Autodesk Inventor part; units mm, degrees
ref_plane "YZ Plane" through (0, 0, 0) normal (1, 0, 0) x (0, 1, 0)
ref_plane "XZ Plane" through (0, 0, 0) normal (0, 1, 0) x (-1, 0, 0)
ref_plane "XY Plane" through (0, 0, 0) normal (0, 0, 1) x (1, 0, 0)
sketch "Sketch1" plane through (0, 0, 0) normal (0, 0, 1) x (1, 0, 0)
  line L0 (0, 0) -> (0, 81.958)
  line L1 (0, 0) -> (0, -81.958)
  line L2 (0, -81.958) -> (-10, -81.958)
  line L3 (-5, -81.958) -> (-5, -67.708) construction
  line L4 (-5, -67.708) -> (-5, -58.708) construction
  line L5 (-10, -81.958) -> (-10, -58.708)
  line L6 (-10, -58.708) -> (0, -58.708)
  line L7 (0, 81.958) -> (-10, 81.958)
  line L8 (-5, 81.958) -> (-5, 66.21) construction
  line L9 (-5, 66.21) -> (-5, 20.031) construction
  line L10 (-5, 20.031) -> (-5, 11.031) construction
  line L11 (-10, 81.958) -> (-10, 11.031)
  line L12 (-10, 11.031) -> (0, 11.031)
  line L13 (0, -58.708) -> (-2, -58.708)
  line L14 (-2, -58.708) -> (-2, 11.031)
  line L15 (0, -81.958) -> (8, -81.958)
  line L16 (8, -81.958) -> (8, 81.958)
  line L17 (8, 81.958) -> (0, 81.958)
  line L18 (0, 81.958) -> (0, -81.958)
  dimension "d0" = 81.958
  dimension "d2" = 163.916
  dimension "d3" = 10
  dimension "d4" = 14.25
  dimension "d5" = 9
  dimension "d6" = 15.748
  dimension "d7" = 46.179
  dimension "d8" = 9
  dimension "d9" = 2
  dimension "d10" = 8
extrude "Extrusion1" add sketch "Sketch1" along normal blind 7
sketch "Sketch2" plane through (0, 0, 0) normal (0, 0, -1) x (-1, 0, 0)
  line L0 (10, 81.958) -> (10, 11.031) construction
  line L1 (10, 46.4945) -> (0, 46.4945) construction
  line L2 (-8, 81.958) -> (10, 81.958)
  line L3 (0, 81.958) -> (-50, 81.958)
  line L4 (-50, 81.958) -> (-50, -81.958)
  line L5 (-50, -81.958) -> (0, -81.958)
  line L6 (0, -81.958) -> (0, 81.958)
  line L7 (-35.1508, -57.5) -> (-20.1508, -57.5)
  line L8 (-20.1508, -57.5) -> (-20.1508, 57.5)
  line L9 (-20.1508, 57.5) -> (-35.1508, 57.5)
  line L10 (-35.1508, 57.5) -> (-35.1508, -57.5)
  line L11 (-35.1508, -57.5) -> (-20.1508, 57.5) construction
  line L12 (-20.1508, -57.5) -> (-35.1508, 57.5) construction
  point P0 (0, 0)
  point P1 (-27.6508, 0)
  dimension "d13" = 10
  dimension "d14" = 50
  dimension "d15" = 15
  dimension "d16" = 115
extrude "Extrusion2" add sketch "Sketch2" along normal blind 9
sketch "Sketch3" plane through (-10, -81.958, 7) normal (0, -1, 0) x (1, 0, 0)
  line L0 (60, -7) -> (18, -7)
  line L1 (60, -7) -> (60, 5)
  line L2 (0, 0) -> (18, 0)
  line L3 (18, 5) -> (18, 0)
  line L4 (60, 5) -> (39, -7)
  line L5 (18, 5) -> (39, -7)
  line L6 (18, -7) -> (18, 0)
  line L7 (18, 0) -> (18, -7)
  point P0 (10, -7)
  dimension "d19" = 12
extrude "Extrusion3" add sketch "Sketch3" against normal up to surface (24.458 mm away)
mirror "Mirror1" about plane through (0, 0, 0) normal (0, 1, 0) of "Extrusion3"
sketch "Sketch4" plane through (0, 0, 7) normal (0, 0, 1) x (1, 0, 0)
  line L0 (-5, -81.958) -> (-5, -67.708) construction
  line L1 (-5, 81.958) -> (-5, 66.21) construction
  line L2 (-5, 66.21) -> (-5, 20.031) construction
  circle A0 centre (-5, -67.708) radius 1.65
  circle A1 centre (-5, 20.031) radius 1.65
  circle A2 centre (-5, 66.21) radius 1.65
  point P0 (0, 0)
  dimension "d22" = 14.25
  dimension "d23" = 46.179
  dimension "d24" = 15.748
  dimension "d25" = 3.3
extrude "Extrusion4" cut sketch "Sketch4" against normal up to surface (7 mm away)
sketch "Sketch5" plane through (0, 0, 7) normal (0, 0, 1) x (1, 0, 0)
  circle A0 centre (-5, -67.708) radius 1.65
  circle A1 centre (-5, -67.708) radius 2.65
  circle A2 centre (-5, 20.031) radius 1.65
  circle A3 centre (-5, 20.031) radius 2.65
  circle A4 centre (-5, 66.21) radius 1.65
  circle A5 centre (-5, 66.21) radius 2.65
  point P0 (0, 0)
  dimension "d28" = 5.3
extrude "Extrusion5" cut sketch "Sketch5" against normal blind 6 contours A0 | A1 | A2 | A3 | A4 | A5
properties part number "Base Extension 2"
Read the model definition and answer for the solid it produces. Units are mm, in the model's axes. A direction names the side the tool comes from. Round coordinates to 2 decimals unless told otherwise and drop trailing zeros. Write each loop counter-clockwise with the first axis right and the second up, starting at its lowest first coordinate (ties: lowest second). Pieces come first, ordered by that corner, then holes. Notation, with made-up numbers: (27, 58) -> (39, 58) arc R25 cw to (39, 74) -> close; hole circle Ø9 at (59, 22). An arc over 180 degrees is marked (long way). Answer in a Markdown table with one row per item. Add a question column.
1) Which of the six approach directions +Z, -Z, +X, -X, +Y, -Y give full straight-line access (tool end or side, diameter ignored) to faces 5 (the face through (1, 1, 7)), 6 (the face through (-3, 19, 0)), 7 (the face through (18.353, -69.9, 6.084)), 8 (the face through (-6, 11.031, 3))?
2) Consider line 1 (Y direction, x = -5, z = 0.3); line 2 (X direction, y = 33.5, z = -2); line 3 (X direction, y = 29, z = 0.5). Determine where each line is inside the solid, lowest interval first.
3) Given P1, Ø4, axis at x = -5, y = 66.21, coming from the -Z side; P2, Ø5.5, axis at y = -69, z = 10, coming from the -X side; P3, Ø4.5, axis at x = 41.5, y = 22, coming from the +Z side; P4, Ø2.5, axis at x = -5, y = 66.21, coming from the +Z side, each flat-ended and moving along its own axis, determine where each tip first touches the part or whether it passes through.
4) Find section D-D, the plane z = 3. Determine the outline of the cut face in (x, y), and give its area (3 significant figures).
5) Find section B-B, the plane z = -6. Determine the outline of the cut face in (x, y).
6) Find section A-A, the plane x = -5. State how many separate pieces and enclosed holes the cut face has, and give its area (3 significant figures).
7) Determine the mould class of faces 1 (the face through (14, 1, 0)), 2 (the face through (50, 1, -3)), 3 (the face through (0, -1, -4)), 4 (the face through (-5.574, 17.444, 4.042)) for opening direction X: pulls with the +X half, pulls with the -X half, needs draft (parallel to the pull), parting line crosses it, or undercut.
8) Find section C-C, the plane y = -20.5. Determine the outline of the cut face in (x, z).
Findings below:
| question | item | result |
|---|---|---|
| 1 | face 5 | +Z, -X, +Y, -Y |
| 1 | face 6 | -Z, -X, +Y, -Y |
| 1 | face 7 | +Z, +Y, -Y |
| 1 | face 8 | +Z, -Z, -X |
| 2 | line 1 | -81.96 to -69.36, -66.06 to -58.71, 11.03 to 18.38, 21.68 to 64.56, 67.86 to 81.96 |
| 2 | line 2 | 0 to 20.15, 35.15 to 50 |
| 2 | line 3 | -10 to 8 |
| 3 | P1 | z = 0 |
| 3 | P2 | x = 8 |
| 3 | P3 | z = 0 |
| 3 | P4 | through |
| 4 | outline | (-10, -81.96) -> (23.75, -81.96) -> (23.75, -57.5) -> (8, -57.5) -> (8, 57.5) -> (23.75, 57.5) -> (23.75, 81.96) -> (-10, 81.96) -> (-10, 11.03) -> (-2, 11.03) -> (-2, -58.71) -> (-10, -58.71) -> close; (34.25, -81.96) -> (50, -81.96) -> (50, -57.5) -> (34.25, -57.5) -> close; (34.25, 57.5) -> (50, 57.5) -> (50, 81.96) -> (34.25, 81.96) -> close; hole circle Ø5.3 at (-5, -67.71); hole circle Ø5.3 at (-5, 20.03); hole circle Ø5.3 at (-5, 66.21) |
| 4 | area | 3,870 mm² |
| 5 | outline | (0, -81.96) -> (50, -81.96) -> (50, 81.96) -> (0, 81.96) -> close; hole (20.15, -57.5) -> (35.15, -57.5) -> (35.15, 57.5) -> (20.15, 57.5) -> close |
| 6 | separate pieces | 5 |
| 6 | enclosed holes | 0 |
| 6 | area | 554 mm² |
| 7 | face 1 | needs draft |
| 7 | face 2 | pulls with the +X half |
| 7 | face 3 | pulls with the -X half |
| 7 | face 4 | undercut |
| 8 | outline | (-2, 0) -> (0, 0) -> (0, -9) -> (20.15, -9) -> (20.15, 0) -> (8, 0) -> (8, 7) -> (-2, 7) -> close; (35.15, -9) -> (50, -9) -> (50, 0) -> (35.15, 0) -> close |
